```python
from build123d import *

# Parameters (mm, degrees)
PAD_DEPTH              = 1.5
SKETCH001_R            = 2.5
POCKET_DEPTH           = 1.501
LINEARPATTERN_COUNT    = 3
LINEARPATTERN_PITCH    = 42.5
LINEARPATTERN001_COUNT = 3
LINEARPATTERN001_PITCH = 42.5


with BuildPart() as part:
    # Sketch → Pad (new body)
    with BuildSketch(Plane.XZ):
        Polygon((0, 0), (100, 0), (100, 15), (15, 15), (15, 100), (0, 100), align=None)
    extrude(amount=PAD_DEPTH)

    # Sketch001 (on Face8 of Pad) → Pocket (cut, through all)
    with BuildSketch(Plane.XZ.offset(1.5)):
        with Locations((7.5, 7.5)):
            Circle(SKETCH001_R)
    pocket = extrude(amount=-POCKET_DEPTH, mode=Mode.SUBTRACT)

    # LinearPattern: Pocket ×3
    with Locations(*[(i * LINEARPATTERN_PITCH, 0, 0) for i in range(1, LINEARPATTERN_COUNT)]):
        add(pocket, mode=Mode.SUBTRACT)

    # LinearPattern001: Pocket ×3
    with Locations(*[(0, 0, i * LINEARPATTERN001_PITCH) for i in range(1, LINEARPATTERN001_COUNT)]):
        add(pocket, mode=Mode.SUBTRACT)


solid = part.part
```
CAD build for the part. Positions are in the model's coordinates, mm. Round coordinates to 2 decimals unless told otherwise and drop trailing zeros. Order: outer loops, then holes, each group sorted by start corner. A loop starts at its lowest first (then second) coordinate and runs counter-clockwise, first axis right, second up. Notation, with made-up numbers: (81, 56.25) - (97, 56.25) arc R11 ccw to (97, 72.25) - close; hole circle Ø9 at (81.5, 26). An arc over 180 degrees is marked (long way). Answer in a Markdown table with one row per item. Add a question column.
(1) Band-saw the part on C-C on z = 7.5. List the corners of the cut face in (x, y), and give its area (4 significant figures).
(2) Band-saw the part on A-A on x = 7.5. List the corners of the cut face in (y, z).
(3) Mould opens along Z. For faces 1 (the face through (8.65, -0.76, 5.28)), 2 (the face through (13, 0, 28)) say: +Z half, -Z half, draft (parallel to the pull), parting line (faces both ways), or undercut.
(4) Band-saw the part on B-B on z = 92.5. List the corners of the cut face in (x, y), and give its area (3 significant figures).
(5) Band-saw the part on D-D on y = -0.75. List the corners of the cut face in (x, z), and give its area (3 significant figures).
(6) Drop a flat-ended pin along its axis: pin 1 Ø0.8 at (x, y) = (55, -1) entering from +Z. Give the stop position or say it passes through.
(7) Probe L1, parallel to Z at x = 7.5, y = -1.15; L2, parallel to X at y = -0.9, z = 74.5; L3, parallel to Z at x = 50, y = -1. List the from-to ranges inside material, lowest first. Write a range as [from, to].
Data:
| question | item | result |
|---|---|---|
| 1 | outline | (0, -1.5) - (5, -1.5) - (5, 0) - (0, 0) - close; (10, -1.5) - (47.5, -1.5) - (47.5, 0) - (10, 0) - close; (52.5, -1.5) - (90, -1.5) - (90, 0) - (52.5, 0) - close; (95, -1.5) - (100, -1.5) - (100, 0) - (95, 0) - close |
| 1 | area | 127.5 mm^2 |
| 2 | outline | (-1.5, 0) - (0, 0) - (0, 5) - (-1.5, 5) - close; (-1.5, 10) - (0, 10) - (0, 47.5) - (-1.5, 47.5) - close; (-1.5, 52.5) - (0, 52.5) - (0, 90) - (-1.5, 90) - close; (-1.5, 95) - (0, 95) - (0, 100) - (-1.5, 100) - close |
| 3 | face 1 | undercut |
| 3 | face 2 | draft |
| 4 | outline | (0, -1.5) - (5, -1.5) - (5, 0) - (0, 0) - close; (10, -1.5) - (15, -1.5) - (15, 0) - (10, 0) - close |
| 4 | area | 15.0 mm^2 |
| 5 | outline | (0, 0) - (100, 0) - (100, 15) - (15, 15) - (15, 100) - (0, 100) - close; hole circle Ø5 at (7.5, 7.5); hole circle Ø5 at (7.5, 50); hole circle Ø5 at (7.5, 92.5); hole circle Ø5 at (50, 7.5); hole circle Ø5 at (92.5, 7.5) |
| 5 | area | 2,680 mm^2 |
| 6 | pin 1 | stops at z = 15 |
| 7 | L1 | z = [0, 5], [10, 47.5], [52.5, 90], [95, 100] |
| 7 | L2 | x = [0, 15] |
| 7 | L3 | z = [0, 5], [10, 15] |
